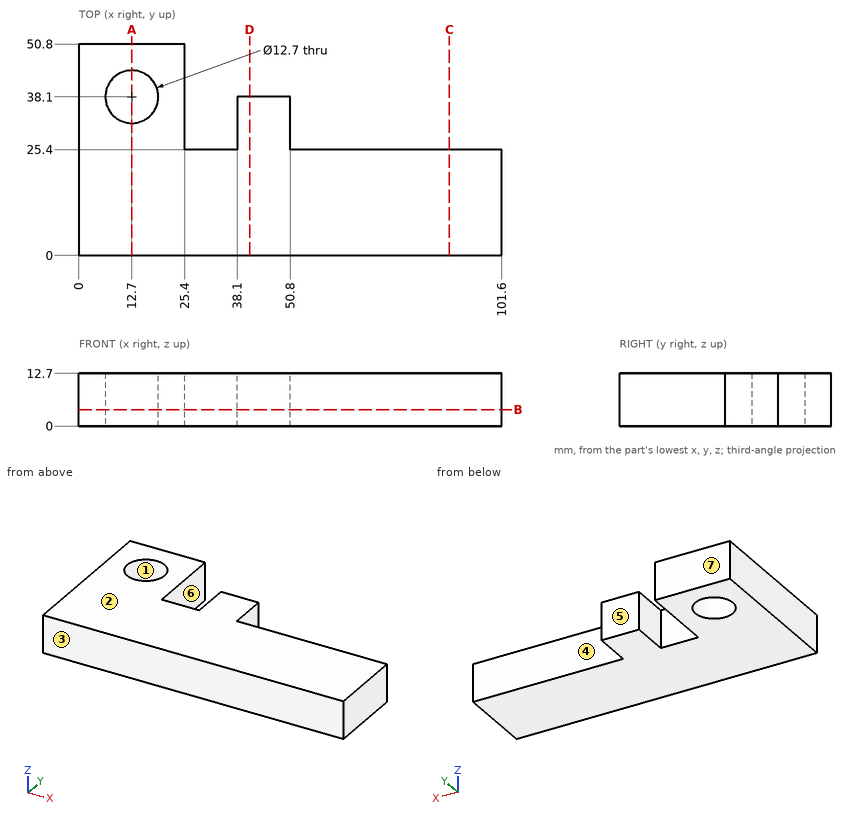
Job drawing, mm, ordinate dimensions from the low corner. One solid piece. A direction names the side the tool comes from. Coordinates: 2 decimals unless noted, no trailing zeros. Write each loop counter-clockwise with the first axis right and the second up, starting at its lowest first coordinate (ties: lowest second). Pieces come first, ordered by that corner, then holes. Notation, with made-up numbers: M 10.25,-20.75 L 55.25,-20.75 A23 cw 55.25,12.25 Z; hole C 11.25,54 d2. An arc over 180 degrees is marked long. Answer as a JSON object with one key per item and string values. Group by question number.
1) Saw through at D-D (x = 41). Write the cut outline in (y, z).
2) Tool access for the marked faces 5, 6 and 7: list every direction of +Z, -Z, +X, -X, +Y, -Y with a clear straight run to the whole face (end or side of a thin tool).
3) Wall check: line 1 (Y direction, x = 95.5, z = 3.5); line 2 (Y direction, x = 12.7, z = 3.75); line 3 (Y direction, x = 11, z = 12.25). Give the ranges that are in metal, low to high. Write a range as from..to.
4) Saw through at C-C (x = 89). Write the cut outline in (y, z).
5) Saw through at B-B (z = 4). Write the cut outline in (x, y), plus the area to 3 significant figures.
6) Pin check, flat tips, straight feed: pin 1 Ø1.5 at (x, z) = (85, 3.5) entering from +Y; pin 2 Ø4 at (y, z) = (33.5, 3.5) entering from +X. Stop position of each tip, or through.
7) Saw through at A-A (x = 12.7). Write the cut outline in (y, z).
8) Mould opens along Y. For the marked faces 1, 2, 3 and 4 say: +Y half, -Y half, draft (parallel to the pull), parting line (faces both ways), or undercut.
Values follow:
{
 "1": {"outline": "M 0,0 L 38.1,0 L 38.1,12.7 L 0,12.7 Z"},
 "2": {"face 5": "+Z, -Z, +X, +Y", "face 6": "+Z, -Z, +Y", "face 7": "+Z, -Z, +X, -X, +Y"},
 "3": {"line 1": "y = 0..25.4", "line 2": "y = 0..31.75, 44.45..50.8", "line 3": "y = 0..31.98, 44.22..50.8"},
 "4": {"outline": "M 0,0 L 25.4,0 L 25.4,12.7 L 0,12.7 Z"},
 "5": {"outline": "M 0,0 L 101.6,0 L 101.6,25.4 L 50.8,25.4 L 50.8,38.1 L 38.1,38.1 L 38.1,25.4 L 25.4,25.4 L 25.4,50.8 L 0,50.8 Z; hole C 12.7,38.1 d12.7", "area": "3,260 mm2"},
 "6": {"pin 1": "stops at y = 25.4", "pin 2": "stops at x = 50.8"},
 "7": {"outline": "M 0,0 L 31.75,0 L 31.75,12.7 L 0,12.7 Z; M 44.45,0 L 50.8,0 L 50.8,12.7 L 44.45,12.7 Z"},
 "8": {"face 1": "undercut", "face 2": "draft", "face 3": "-Y half", "face 4": "+Y half"}
}
